from build123d import *

# Parameters (mm, degrees)
F0_R     = 2.4
F1_DEPTH = 150


# Not quite as in the source:
# - a feature names something its author has since deleted; it is built from what else it names


with BuildPart() as f1:
    # F0 (on Top) → F1 (new body)
    with BuildSketch(Plane.XY):
        with BuildLine():
            ThreePointArc((11.8809631136, -1.6860354369), (11.9702037861, -0.8451161569), (12, 0))
            ThreePointArc((12, 0), (11.4820297491, 3.4875482565), (9.9728345264, 6.6740221388))
            Line((9.9728345264, 6.6740221388), (8.7545372195, 5.7024624569))
            Line((8.7545372195, 5.7024624569), (9.1286311006, 5.2333635674))
            Line((9.1286311006, 5.2333635674), (6.1566837752, 2.2237906583))
            Line((6.1566837752, 2.2237906583), (3.5380266074, 5.5074828847))
            Line((3.5380266074, 5.5074828847), (7.1334637347, 7.7352243113))
            Line((7.1334637347, 7.7352243113), (7.5075576158, 7.2661254218))
            Line((7.5075576158, 7.2661254218), (8.7258549227, 8.2376851038))
            ThreePointArc((8.7258549227, 8.2376851038), (5.2066048694, 10.8116264148), (1, 11.9582607431))
            Line((1, 11.9582607431), (1, 10.4))
            Line((1, 10.4), (1.6, 10.4))
            Line((1.6, 10.4), (2.1, 6.2))
            Line((2.1, 6.2), (-2.1, 6.2))
            Line((-2.1, 6.2), (-1.6, 10.4))
            Line((-1.6, 10.4), (-1, 10.4))
            Line((-1, 10.4), (-1, 11.9582607431))
            ThreePointArc((-1, 11.9582607431), (-5.2066048694, 10.8116264148), (-8.7258549227, 8.2376851038))
            Line((-8.7258549227, 8.2376851038), (-7.5075576158, 7.2661254218))
            Line((-7.5075576158, 7.2661254218), (-7.1334637347, 7.7352243113))
            Line((-7.1334637347, 7.7352243113), (-3.5380266074, 5.5074828847))
            Line((-3.5380266074, 5.5074828847), (-6.1566837752, 2.2237906583))
            Line((-6.1566837752, 2.2237906583), (-9.1286311006, 5.2333635674))
            Line((-9.1286311006, 5.2333635674), (-8.7545372195, 5.7024624569))
            Line((-8.7545372195, 5.7024624569), (-9.9728345264, 6.6740221388))
            ThreePointArc((-9.9728345264, 6.6740221388), (-11.6991349462, 2.6702512075), (-11.8809631136, -1.6860354369))
            Line((-11.8809631136, -1.6860354369), (-10.3617712206, -1.339289801))
            Line((-10.3617712206, -1.339289801), (-10.495283781, -0.7543330537))
            Line((-10.495283781, -0.7543330537), (-6.5118470168, 0.6677188251))
            Line((-6.5118470168, 0.6677188251), (-5.5772590942, -3.4269784061))
            Line((-5.5772590942, -3.4269784061), (-9.7832167924, -3.8741023726))
            Line((-9.7832167924, -3.8741023726), (-9.9167293527, -3.2891456253))
            Line((-9.9167293527, -3.2891456253), (-11.4359212456, -3.6358912612))
            ThreePointArc((-11.4359212456, -3.6358912612), (-9.3819777896, -7.4818776223), (-6.0894637525, -10.3401369047))
            Line((-6.0894637525, -10.3401369047), (-5.4133597547, -8.9361924871))
            Line((-5.4133597547, -8.9361924871), (-5.9539410755, -8.6758622436))
            Line((-5.9539410755, -8.6758622436), (-4.5821138051, -4.6748511288))
            Line((-4.5821138051, -4.6748511288), (-0.7980445599, -6.4971628331))
            Line((-0.7980445599, -6.4971628331), (-3.0708406982, -10.0642902088))
            Line((-3.0708406982, -10.0642902088), (-3.6114220189, -9.8039599653))
            Line((-3.6114220189, -9.8039599653), (-4.2875260167, -11.2079043829))
            ThreePointArc((-4.2875260167, -11.2079043829), (0, -12), (4.2875260167, -11.2079043829))
            Line((4.2875260167, -11.2079043829), (3.6114220189, -9.8039599653))
            Line((3.6114220189, -9.8039599653), (3.0708406982, -10.0642902088))
            Line((3.0708406982, -10.0642902088), (0.7980445599, -6.4971628331))
            Line((0.7980445599, -6.4971628331), (4.5821138051, -4.6748511288))
            Line((4.5821138051, -4.6748511288), (5.9539410755, -8.6758622436))
            Line((5.9539410755, -8.6758622436), (5.4133597547, -8.9361924871))
            Line((5.4133597547, -8.9361924871), (6.0894637525, -10.3401369047))
            ThreePointArc((6.0894637525, -10.3401369047), (9.3819777896, -7.4818776223), (11.4359212456, -3.6358912612))
            Line((11.4359212456, -3.6358912612), (9.9167293527, -3.2891456253))
            Line((9.9167293527, -3.2891456253), (9.7832167924, -3.8741023726))
            Line((9.7832167924, -3.8741023726), (5.5772590942, -3.4269784061))
            Line((5.5772590942, -3.4269784061), (6.5118470168, 0.6677188251))
            Line((6.5118470168, 0.6677188251), (10.495283781, -0.7543330537))
            Line((10.495283781, -0.7543330537), (10.3617712206, -1.339289801))
            Line((10.3617712206, -1.339289801), (11.8809631136, -1.6860354369))
        make_face()
        Circle(F0_R, mode=Mode.SUBTRACT)
    extrude(amount=F1_DEPTH)


solid = f1.part
Build history of the part. All positions in model axes, mm. A direction names the side the tool comes from. Give positions to 0.01 mm unless a question says otherwise; leave off trailing zeros. Answer in a Markdown table with one row per item.
Item 1: Flat gauge pins, fed straight in: P1, Ø3.5, axis at x = -0.5, z = 109.5, coming from the +Y side; P2, Ø0.5, axis at y = 11, z = 83.5, coming from the -X side; P3, Ø1, axis at y = -9.5, z = 98, coming from the -X side; P4, Ø10, axis at y = 7, z = 16.5, coming from the +X side. Where does each tip first touch, or does it go through?
Findings below:
| item | result |
|---|---|
| P1 | stops at y = 11.96 |
| P2 | stops at x = -5.33 |
| P3 | stops at x = -7.94 |
| P4 | stops at x = 11.83 |
Item 2: Mould opens along X. For faces 3 (the cylindrical face through (0, -12, 74)), 4 (the flat face through (5.26, -6.65, 73.95)), 5 (the flat face through (0, 3, 0)), 6 (the flat face through (-8.531, -0.053, 73.95)) say: pulls with the +X half, pulls with the -X half, needs draft (parallel to the pull), parting line crosses it, or undercut.
Findings below:
| item | result |
|---|---|
| face 3 | parting line crosses it |
| face 4 | undercut |
| face 5 | needs draft |
| face 6 | undercut |
Item 3: Probe line 1 along Y through (x, z) = (0, 41.5); line 2 along X through (y, z) = (6.5, 45.5); line 3 along Y through (x, z) = (8.5, 77). List the from-to ranges inside material, lowest first. Write a range as [from, to].
Findings below:
| item | result |
|---|---|
| line 1 | y = [-12, -2.4], [2.4, 6.2] |
| line 2 | x = [-10.09, -9.75], [-5.14, -2.06], [2.06, 5.14], [9.75, 10.09] |
| line 3 | y = [-8.47, -3.74], [-0.04, 4.6], [8.06, 8.47] |
Item 4: Tool access for faces 1 (the flat face through (4.9, 3.8, 74)), 2 (the cylindrical face through (-5.15, 10.84, 73.95)): list every direction of +Z, -Z, +X, -X, +Y, -Y with a clear straight run to the whole face (end or side of a thin tool).
Findings below:
| item | result |
|---|---|
| face 1 | +Z, -Z |
| face 2 | +Z, -Z, -X, +Y |
